```python
from build123d import *

# Parameters (mm, degrees)
F0_R     = 1
F0_R_2   = 0.5
F0_W     = 24
F0_H     = 13.5
F1_DEPTH = 3
F3_R     = 3


with BuildPart() as f1:
    # F0 (on Top) → F1 (new body)
    with BuildSketch(Plane.XY):
        Polygon((20, -8.5), (20, 12.5), (16, 12.5), (-20, 12.5), (-20, -8.5), (-20, -12.5), (-16, -12.5), (16, -12.5), (20, -12.5), align=None)
        with Locations((-16, -8.5)):
            Circle(F0_R, mode=Mode.SUBTRACT)
        with Locations((16, -8.5)):
            Circle(F0_R, mode=Mode.SUBTRACT)
        with Locations((-13.75, 0)):
            Circle(F0_R_2, mode=Mode.SUBTRACT)
        with Locations((-16, 8.5)):
            Circle(F0_R, mode=Mode.SUBTRACT)
        Rectangle(F0_W, F0_H, mode=Mode.SUBTRACT)
        with Locations((13.75, 0)):
            Circle(F0_R_2, mode=Mode.SUBTRACT)
        with Locations((16, 8.5)):
            Circle(F0_R, mode=Mode.SUBTRACT)
    extrude(amount=F1_DEPTH)

    # F2: F1 across face


with BuildPart() as f1_1:
    add(f1.part)
    add(f1.part.mirror(Plane(origin=(0, -12.5, 1.5), x_dir=(1, 0, 0), z_dir=(0, -1, 0))))

    # F3
    f3_edges = [f1_1.edges().sort_by_distance(p)[0] for p in [
        (-20, -37.5, 1.5),
        (20, -37.5, 1.5),
        (20, 12.5, 1.5),
        (-20, 12.5, 1.5),
    ]]
    fillet(f3_edges, radius=F3_R)


solid = f1_1.part
```
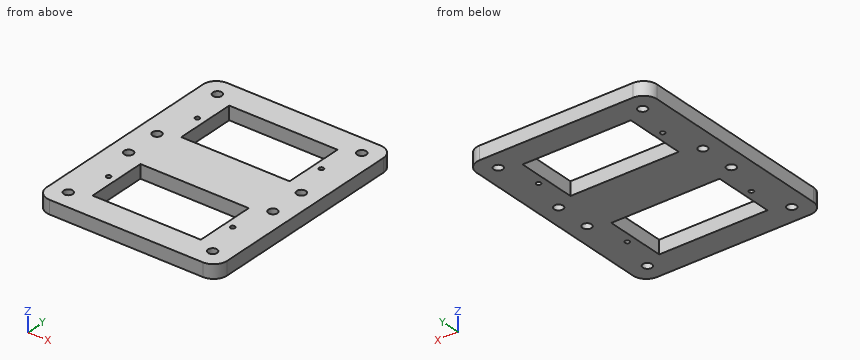
Model file for the job. Use its own axes, mm. Coordinates: 2 decimals unless noted, no trailing zeros. Loops run counter-clockwise (first coordinate to the right, second up) from the corner with the lowest first, then second, coordinate; pieces in that order, holes last. Notation, with made-up numbers: M 78,-3.75 L 91,-3.75 A11 cw 91,1.25 Z; hole C 7.25,35 d1. An arc over 180 degrees is marked long. Use CSV: the item, a comma, the result in double quotes. Start each with the question number.
1. Band-saw the part on A-A, the plane y = -33.5. List the corners of the cut face in (x, z), then the cut area to 3 significant figures.
2. Band-saw the part on D-D, the plane x = 16. List the corners of the cut face in (y, z), then the cut area to 3 significant figures.
3. Band-saw the part on C-C, the plane z = 1.1. Give the number of separate pieces and of enclosed holes in the cut face, then the cut area to 3 significant figures.
4. Band-saw the part on B-B, the plane x = 6.5. List the corners of the cut face in (y, z).
5. Probe probe 1 along Y at (x, z) = (16, 1.7); probe 2 along Y at (x, z) = (-5.5, 0.9); probe 3 along X at (y, z) = (-2.5, 2.7). List the from-to ranges inside material, lowest first. Write a range as [from, to].
Entries:
1,outline,"M -20,0 L -17,0 L -17,3 L -20,3 Z; M -15,0 L 15,0 L 15,3 L -15,3 Z; M 17,0 L 20,0 L 20,3 L 17,3 Z"
1,area,"108 mm2"
2,outline,"M -37.5,0 L -34.5,0 L -34.5,3 L -37.5,3 Z; M -32.5,0 L -17.5,0 L -17.5,3 L -32.5,3 Z; M -15.5,0 L -9.5,0 L -9.5,3 L -15.5,3 Z; M -7.5,0 L 7.5,0 L 7.5,3 L -7.5,3 Z; M 9.5,0 L 12.5,0 L 12.5,3 L 9.5,3 Z"
2,area,"126 mm2"
3,separate pieces,"1"
3,enclosed holes,"14"
3,area,"1,320 mm2"
4,outline,"M -37.5,0 L -31.75,0 L -31.75,3 L -37.5,3 Z; M -18.25,0 L -6.75,0 L -6.75,3 L -18.25,3 Z; M 6.75,0 L 12.5,0 L 12.5,3 L 6.75,3 Z"
5,probe 1,"y = [-37.5, -34.5], [-32.5, -17.5], [-15.5, -9.5], [-7.5, 7.5], [9.5, 12.5]"
5,probe 2,"y = [-37.5, -31.75], [-18.25, -6.75], [6.75, 12.5]"
5,probe 3,"x = [-20, -12], [12, 20]"
